Autodesk Inventor part; units mm, degrees
ref_plane "YZ Plane" through (0, 0, 0) normal (1, 0, 0) x (0, 1, 0)
ref_plane "XZ Plane" through (0, 0, 0) normal (0, 1, 0) x (-1, 0, 0)
ref_plane "XY Plane" through (0, 0, 0) normal (0, 0, 1) x (1, 0, 0)
sketch "Sketch1" plane through (0, 0, 0) normal (1, 0, 0) x (0, 1, 0)
  circle A0 centre (0, 0) radius 1.75
  circle A1 centre (0, 0) radius 2.5
  dimension "d0" = 3.5
  dimension "d1" = 5
extrude "Extrusion1" add sketch "Sketch1" along normal blind 3.5
sketch "Sketch2" plane through (3.5, 0, 0) normal (1, 0, 0) x (0, 0, -1)
  circle A0 centre (0, 0) radius 2.5 construction
  line L0 (0, 2.5) -> (0, 2.375) construction
  line L1 (0, 2.375) -> (0.25, 2.375) construction
  line L2 (0.25, 2.375) -> (-0.25, 2.375) construction
  line L3 (-0.25, 2.375) -> (0.25, 2.375)
  line L4 (0, 2.375) -> (-0.5, 2.375)
  line L5 (-0.5, 2.375) -> (0.5, 2.375)
  line L6 (0, 2.375) -> (0, 3.875) construction
  line L7 (0, 3.875) -> (1, 3.875) construction
  line L8 (0, 3.875) -> (1, 3.875)
  line L9 (0, 3.875) -> (-0.5, 2.375)
  arc A1 (1, 3.875) -> (0.5, 2.375) centre (1.158, 2.989) ccw
  line L10 (0, 3.875) -> (1.5, 3.875)
  line L11 (1.5, 3.875) -> (1.5, 4)
  line L12 (1.5, 4) -> (0, 4)
  line L13 (0, 4) -> (0, 3.875)
  dimension "d4" = 0.125
  dimension "d5" = 0.25
  dimension "d6" = 0.5
  dimension "d11" = 0.5
  dimension "d12" = 1
  dimension "d14" = 1
  dimension "d15" = 0.9
  dimension "d16" = 1.5
  dimension "d17" = 0.125
extrude "Extrusion2" add sketch "Sketch2" against normal blind 3.5
fillet "Fillet1" radius 2 1 edges at (1.75, 3.875, 0)
pattern_circular "Circular Pattern1" count 6 over 360 about axis through (0, 0, 0) along (1, 0, 0) of "Extrusion2"
properties part number "mtv_gear6_1-15"
The listing builds one solid part. Answer for the finished solid, in the listing's coordinates (mm). A direction names the side the tool comes from. Coordinates: 2 decimals unless noted, no trailing zeros. Loops run counter-clockwise (first coordinate to the right, second up) from the corner with the lowest first, then second, coordinate; pieces in that order, holes last. Notation, with made-up numbers: (-0.5, 23.5) -> (30.5, 23.5) arc R24 ccw to (30.5, 56.5) -> close; hole circle Ø1 at (60.5, 77). An arc over 180 degrees is marked (long way). Answer in a Markdown table with one row per item. Add a question column.
1. The part is cut by section C-C, the plane y = 1.25. Write down the section's boundary in (x, z), then the cut area to 3 significant figures.
2. The part is cut by section B-B, the plane z = -1.25. Write down the section's boundary in (x, y) (3 decimals).
3. For faces 1 (the flat face through (1.774, -1.341, 3.844)), 2 (the cylindrical face through (1.726, 2.147, 1.28)), 3 (the flat face through (1.77, -1.39, -2.87)), 4 (the cylindrical face through (1.774, 1.385, -3.056)), 5 (the cylindrical face through (1.726, -2.147, -1.28)), determine the directions among +Z, -Z, +X, -X, +Y, -Y from which every point of the face is accessible in a straight line to the end or side of a thin tool.
4. The part is cut by section D-D, the plane y = -1.5. Write down the section's boundary in (x, z), then the cut area to 3 significant figures.
5. Flat-ended cylindrical pins translate along their axes: P1, Ø0.6, axis at x = 2, z = 1, coming from the +Y side; P2, Ø4, axis at y = -1.5, z = 0.5, coming from the -X side; P3, Ø2, axis at y = 0, z = 0, coming from the -X side. Find the tip coordinate at first contact, or state that the pin passes through.
6. Consider line 1 (Z direction, x = 2.6, y = 0); line 2 (Y direction, x = 1.45, z = -2.75); line 3 (Z direction, x = 2.85, y = 2.5). Determine where each line is inside the solid, lowest interval first. Write a range as [from, to].
7. The part is cut by section A-A, the plane y = 0. Write down the section's boundary in (x, z), then the cut area to 3 significant figures.
8. Determine the mould class of faces 6 (the cylindrical face through (1.774, 1.954, 2.727)), 7 (the flat face through (1.77, -1.79, 2.63)), 8 (the flat face through (1.77, 1.79, -2.63)), 9 (the flat face through (1.77, 1.39, 2.87)) for opening direction Y: +Y half, -Y half, draft (parallel to the pull), parting line (faces both ways), or undercut.
Answer below:
| question | item | result |
|---|---|---|
| 1 | outline | (0, -3.9) -> (3.5, -3.9) -> (3.5, -3.65) -> (0, -3.65) -> close; (0, -2.68) -> (3.5, -2.68) -> (3.5, -1.22) -> (0, -1.22) -> close; (0, 1.22) -> (3.5, 1.22) -> (3.5, 2.75) -> (0, 2.75) -> close |
| 1 | area | 11.3 mm2 |
| 2 | outline | (0, -2.165) -> (3.5, -2.165) -> (3.5, -1.225) -> (0, -1.225) -> close; (0, 1.225) -> (3.5, 1.225) -> (3.5, 2.165) -> (0, 2.165) -> close; (0, 3.875) -> (3.5, 3.875) -> (3.5, 4) -> (0, 4) -> close |
| 3 | face 1 | +Z, +X, -X, -Y |
| 3 | face 2 | +X, -X, +Y |
| 3 | face 3 | -Z, +X, -X |
| 3 | face 4 | +X, -X |
| 3 | face 5 | +X, -X, -Y |
| 4 | outline | (0, -2.97) -> (3.5, -2.97) -> (3.5, -0.9) -> (0, -0.9) -> close; (0, 0.9) -> (3.5, 0.9) -> (3.5, 3.75) -> (0, 3.75) -> close |
| 4 | area | 17.2 mm2 |
| 5 | P1 | y = 2.4 |
| 5 | P2 | x = 0 |
| 5 | P3 | through |
| 6 | line 1 | [-2.5, -1.75], [1.75, 2.5] |
| 6 | line 2 | [-3.24, -2.99], [-1.99, -1.25], [1.29, 1.81] |
| 6 | line 3 | [-0.4, 0.46], [2.91, 3.18] |
| 7 | outline | (0, -2.5) -> (3.5, -2.5) -> (3.5, -1.75) -> (0, -1.75) -> close; (0, 1.75) -> (3.5, 1.75) -> (3.5, 2.5) -> (0, 2.5) -> close |
| 7 | area | 5.25 mm2 |
| 8 | face 6 | undercut |
| 8 | face 7 | -Y half |
| 8 | face 8 | +Y half |
| 8 | face 9 | undercut |
